Work out the finished part from the listing and answer in its coordinate system (mm). A direction names the side the tool comes from. Round coordinates to 2 decimals unless told otherwise and drop trailing zeros. Loops run counter-clockwise (first coordinate to the right, second up) from the corner with the lowest first, then second, coordinate; pieces in that order, holes last. Notation, with made-up numbers: M 51.5,0 L 69.5,0 A6 ccw 69.5,10 Z; hole C 71,-14.5 d5. An arc over 180 degrees is marked long. One line per item, written item: value.
```python
from build123d import *

# Parameters (mm, degrees)
BOSS_EXTRUDE1_DEPTH      = 2.38125
M3_CLEARANCE_HOLE1_D     = 3.6
M3_CLEARANCE_HOLE1_DEPTH = 10
M3_CLEARANCE_HOLE1_TIP   = 1.081549114
SKETCH5_W                = 120
SKETCH5_H                = 4.7625
CUT_EXTRUDE1_DEPTH       = 10
SKETCH6_R                = 2
CUT_EXTRUDE2_DEPTH       = 10
SKETCH7_W                = 70
SKETCH7_H                = 50
CUT_EXTRUDE3_DEPTH       = 10
FILLET1_R                = 20
FILLET2_R                = 5


with BuildPart() as part:
    # Sketch1 → Boss-Extrude1 (new, symmetric)
    with BuildSketch(Plane(origin=(0, 0, 0), x_dir=(1, 0, 0), z_dir=(0, 1, 0))):
        Polygon((-200, 90), (-160, 90), (-160, 50), (-70, 50), (-70, 90), (70, 90), (70, 50), (160, 50), (160, 90), (200, 90), (200, -90), (160, -90), (160, -50), (70, -50), (70, -90), (-70, -90), (-70, -50), (-160, -50), (-160, -90), (-200, -90), align=None)
    extrude(amount=BOSS_EXTRUDE1_DEPTH, both=True)

    # M3 Clearance Hole1
    with Locations(Plane(origin=(0, 2.38125, 0), x_dir=(1, 0, 0), z_dir=(0, 1, 0))):
        with Locations((135, -35), (85, -35), (85, 35), (135, 35)):
            Hole(M3_CLEARANCE_HOLE1_D / 2, depth=M3_CLEARANCE_HOLE1_DEPTH)
            with Locations((0, 0, -(M3_CLEARANCE_HOLE1_DEPTH + M3_CLEARANCE_HOLE1_TIP / 2))):  # 118° drill point
                Cone(0, M3_CLEARANCE_HOLE1_D / 2, M3_CLEARANCE_HOLE1_TIP, mode=Mode.SUBTRACT)

    # Sketch5 → Cut-Extrude1 (cut)
    with BuildSketch(Plane(origin=(0, 2.38125, 0), x_dir=(1, 0, 0), z_dir=(0, 1, 0))):
        with Locations((0, 82.85625)):
            Rectangle(SKETCH5_W, SKETCH5_H)
        with Locations((0, -82.85625)):
            Rectangle(SKETCH5_W, SKETCH5_H)
    extrude(amount=-CUT_EXTRUDE1_DEPTH, mode=Mode.SUBTRACT)

    # Sketch6 → Cut-Extrude2 (cut)
    with BuildSketch(Plane.XZ.offset(2.38125)):
        with Locations(Location((-166, 84, 0), (0, 0, 270))):
            Circle(SKETCH6_R)
        with Locations(Location((-166, 64.5, 0), (0, 0, 270))):
            Circle(SKETCH6_R)
        with Locations(Location((-64, 84, 0), (0, 0, 270))):
            Circle(SKETCH6_R)
        with Locations(Location((-64, 64.5, 0), (0, 0, 270))):
            Circle(SKETCH6_R)
        with Locations(Location((-166, -64.5, 0), (0, 0, 270))):
            Circle(SKETCH6_R)
        with Locations(Location((-166, -84, 0), (0, 0, 270))):
            Circle(SKETCH6_R)
        with Locations(Location((-64, -64.5, 0), (0, 0, 270))):
            Circle(SKETCH6_R)
        with Locations(Location((-64, -84, 0), (0, 0, 270))):
            Circle(SKETCH6_R)
    cut_extrude2 = extrude(amount=-CUT_EXTRUDE2_DEPTH, mode=Mode.SUBTRACT)

    # Mirror1: Cut-Extrude2 across plane
    add(cut_extrude2.mirror(Plane.ZY), mode=Mode.SUBTRACT)

    # Sketch7 → Cut-Extrude3 (cut)
    with BuildSketch(Plane(origin=(0, 2.38125, 0), x_dir=(1, 0, 0), z_dir=(0, 1, 0))):
        with Locations((110, 0)):
            Rectangle(SKETCH7_W, SKETCH7_H)
    extrude(amount=-CUT_EXTRUDE3_DEPTH, mode=Mode.SUBTRACT)

    # Fillet1
    fillet1_edges = [part.edges().sort_by_distance(p)[0] for p in [
        (75, 0, 25),
        (75, 0, -25),
        (145, 0, -25),
        (145, 0, 25),
        (-200, 0, -90),
        (200, 0, -90),
        (200, 0, 90),
        (-200, 0, 90),
    ]]
    fillet(fillet1_edges, radius=FILLET1_R)

    # Fillet2
    fillet2_edges = [part.edges().sort_by_distance(p)[0] for p in [
        (-160, 0, -50),
        (-70, 0, -50),
        (70, 0, -50),
        (160, 0, -50),
        (160, 0, 50),
        (70, 0, 50),
        (-70, 0, 50),
        (-160, 0, 50),
    ]]
    fillet(fillet2_edges, radius=FILLET2_R)


solid = part.part
```
1) Find section A-A (x = 6.5). Give the vertices of the cut face in (y, z) (1 decimal), then the cut area to 3 significant figures.
Check values:
outline: M -2.4,-90 L 2.4,-90 L 2.4,-85.2 L -2.4,-85.2 Z; M -2.4,-80.5 L 2.4,-80.5 L 2.4,80.5 L -2.4,80.5 Z; M -2.4,85.2 L 2.4,85.2 L 2.4,90 L -2.4,90 Z
area: 812 mm2
2) The mould has two halves that part along Z. Classify faces 1 (the face through (194.297, -0.033, 83.986)), 2 (the face through (139.297, -0.033, 18.986)), 3 (the face through (3, -2.381, -1)): +Z half, -Z half, draft (parallel to the pull), parting line (faces both ways), or undercut.
Check values:
face 1: +Z half
face 2: undercut
face 3: draft
3) Find section B-B (y = 1.6). Give the number of separate pieces and of enclosed holes in the cut face, then the cut area to 3 significant figures.
Check values:
separate pieces: 1
enclosed holes: 23
area: 52,800 mm2
4) For faces 4 (the face through (-194.297, 0.033, 83.986)), 5 (the face through (81.014, -0.033, 19.297)), determine the directions among +Z, -Z, +X, -X, +Y, -Y from which every point of the face is accessible in a straight line to the end or side of a thin tool.
Check values:
face 4: +Z, -X, +Y, -Y
face 5: +Y, -Y
5) Find the intervals of material crossed by probe 1 along Z at (x, y) = (10, 2) (1 decimal); probe 2 along Z at (x, y) = (64, 0.9); probe 3 along X at (y, z) = (1.15, 34.5), in increasing order. Write a range as from..to.
Check values:
probe 1: -90..-85.2, -80.5..80.5, 85.2..90
probe 2: -90..-86, -82..-66.5, -62.5..62.5, 66.5..82, 86..90
probe 3: -200..83.27, 86.73..133.27, 136.73..200
6) Find section C-C (x = -126). Give the vertices of the cut face in (y, z), then the cut area to 3 significant figures.
Check values:
outline: M -2.38,-50 L 2.38,-50 L 2.38,50 L -2.38,50 Z
area: 476 mm2
7) This flat-tipped pin is pushed along its axis until it touches: pin 1 (1.4 mm diameter, centred on x = 110, y = 0.5, fed in from +Z). Where does it stop, or does it pass through?
Check values:
pin 1: z = 50
